```python
from build123d import *

# Parameters (mm, degrees)
SKETCH_1_W      = 65
SKETCH_1_H      = 55
SKETCH_1_R      = 1.5
EXTRUDE_1_DEPTH = 4


with BuildPart() as part:
    # 草图1 → 凸台-拉伸1 (new body)
    with BuildSketch(Plane.XY):
        Rectangle(SKETCH_1_W, SKETCH_1_H)
        with Locations((-21.5, 14.5)):
            Circle(SKETCH_1_R, mode=Mode.SUBTRACT)
        with Locations((-21.5, -14.5)):
            Circle(SKETCH_1_R, mode=Mode.SUBTRACT)
        with Locations((16.5, 23.5)):
            Circle(SKETCH_1_R, mode=Mode.SUBTRACT)
        with Locations((25.5, 23.5)):
            Circle(SKETCH_1_R, mode=Mode.SUBTRACT)
        with Locations((16.5, -23.5)):
            Circle(SKETCH_1_R, mode=Mode.SUBTRACT)
        with Locations((25.5, -23.5)):
            Circle(SKETCH_1_R, mode=Mode.SUBTRACT)
        Polygon((23.5, -19.5), (23.5, 19.5), (-18.5, 19.5), (-18.5, 11.5), (-26.5, 11.5), (-26.5, -11.5), (-18.5, -11.5), (-18.5, -19.5), align=None, mode=Mode.SUBTRACT)
    extrude(amount=EXTRUDE_1_DEPTH)


solid = part.part
```
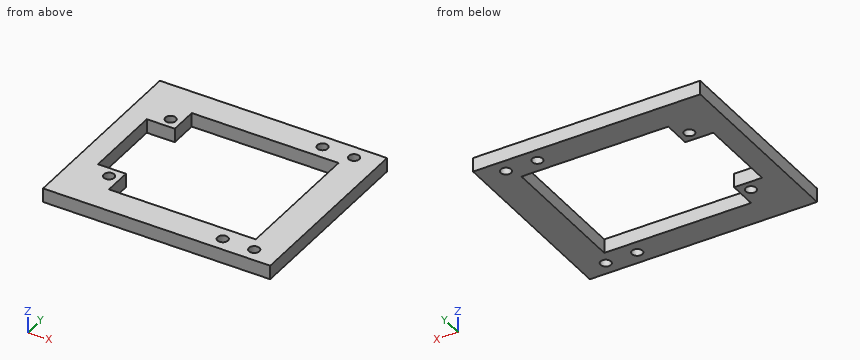
Build history of the part. All positions in model axes, mm. Coordinates: 2 decimals unless noted, no trailing zeros. Order: outer loops, then holes, each group sorted by start corner. A loop starts at its lowest first (then second) coordinate and runs counter-clockwise, first axis right, second up. Notation, with made-up numbers: M 54.25,18 L 64.25,18 A19 ccw 64.25,50 Z; hole C 84.25,-8 d9. An arc over 180 degrees is marked long. One line per question, with ' | ' between items. Start each with the question number.
1. Wall check: line 1 along Y through (x, z) = (16.5, 1.7); line 2 along Y through (x, z) = (-21.5, 2.45); line 3 along X through (y, z) = (-12, 3.4). Give the ranges that are in metal, low to high. Write a range as [from, to].
2. Cut at B-B (x = 3). Write the cut outline in (y, z), plus the area to 3 significant figures.
3. Cut at A-A (y = -2.5). Write the cut outline in (x, z), plus the area to 3 significant figures.
4. Cut at D-D (z = 2.1). Write the cut outline in (x, y).
5. Cut at C-C (y = 23.5). Write the cut outline in (x, z), plus the area to 3 significant figures.
The answers:
1) line 1: y = [-27.5, -25], [-22, -19.5], [19.5, 22], [25, 27.5] | line 2: y = [-27.5, -16], [-13, -11.5], [11.5, 13], [16, 27.5] | line 3: x = [-32.5, -18.5], [23.5, 32.5]
2) outline: M -27.5,0 L -19.5,0 L -19.5,4 L -27.5,4 Z; M 19.5,0 L 27.5,0 L 27.5,4 L 19.5,4 Z | area: 64.0 mm2
3) outline: M -32.5,0 L -26.5,0 L -26.5,4 L -32.5,4 Z; M 23.5,0 L 32.5,0 L 32.5,4 L 23.5,4 Z | area: 60.0 mm2
4) outline: M -32.5,-27.5 L 32.5,-27.5 L 32.5,27.5 L -32.5,27.5 Z; hole M -26.5,-11.5 L -18.5,-11.5 L -18.5,-19.5 L 23.5,-19.5 L 23.5,19.5 L -18.5,19.5 L -18.5,11.5 L -26.5,11.5 Z; hole C -21.5,-14.5 d3; hole C -21.5,14.5 d3; hole C 16.5,-23.5 d3; hole C 16.5,23.5 d3; hole C 25.5,-23.5 d3; hole C 25.5,23.5 d3
5) outline: M -32.5,0 L 15,0 L 15,4 L -32.5,4 Z; M 18,0 L 24,0 L 24,4 L 18,4 Z; M 27,0 L 32.5,0 L 32.5,4 L 27,4 Z | area: 236 mm2
